Source: CAD feature listing. Evaluate the final solid. Frame: model axes, mm. A direction names the side the tool comes from. Round coordinates to 2 decimals unless told otherwise and drop trailing zeros. Loops run counter-clockwise (first coordinate to the right, second up) from the corner with the lowest first, then second, coordinate; pieces in that order, holes last. Notation, with made-up numbers: M 7.5,63 L 60.5,63 A27 cw 60.5,93 Z; hole C 78.25,54 d8. An arc over 180 degrees is marked long. One line per item, written item: value.
from build123d import *

# Parameters (mm, degrees)
SKETCH1_W           = 20
SKETCH1_H           = 6
BOSS_EXTRUDE1_DEPTH = 30
SKETCH2_W           = 40
SKETCH2_H           = 40
BOSS_EXTRUDE2_DEPTH = 20
FILLET1_R           = 10


with BuildPart() as part:
    # Sketch1 → Boss-Extrude1 (new body)
    with BuildSketch(Plane.XY):
        with Locations((-20, -3)):
            Rectangle(SKETCH1_W, SKETCH1_H)
    extrude(amount=BOSS_EXTRUDE1_DEPTH)

    # Sketch2 → Boss-Extrude2 (add)
    with BuildSketch(Plane.XY):
        with Locations((-10, 14)):
            Rectangle(SKETCH2_W, SKETCH2_H)
    extrude(amount=-BOSS_EXTRUDE2_DEPTH)

    # Fillet1
    # the kernel refuses this fillet: 10 mm, written as the material it adds along each edge
    with BuildSketch(Plane(origin=(-10, 0, 0), x_dir=(0, 1, 0), z_dir=(-1, 0, 0))) as fillet1_piece_1:
        with BuildLine():
            CenterArc((FILLET1_R, -FILLET1_R), FILLET1_R, 90, 90)
            Line((0, -FILLET1_R), (0, 0))
            Line((0, 0), (FILLET1_R, 0))
        make_face()
    extrude(amount=20)
    # the kernel refuses this fillet: 10 mm, written as the material it takes off along each edge
    with BuildSketch(Plane(origin=(10, 34, 25), x_dir=(-1, 0, 0), z_dir=(0, 0, -1))) as fillet1_2_piece_1:
        with BuildLine():
            CenterArc((FILLET1_R, -FILLET1_R), FILLET1_R, 90, 90)
            Line((0, -FILLET1_R), (0, 0))
            Line((0, 0), (FILLET1_R, 0))
        make_face()
    extrude(amount=70, mode=Mode.SUBTRACT)
    with BuildSketch(Plane(origin=(12.912878475, 0, 30), x_dir=(0, 0, -1), z_dir=(-1, 0, 0))) as fillet1_2_piece_2:
        with BuildLine():
            CenterArc((9.16515139, 10), FILLET1_R, 203.578178478, 66.421821522)
            Line((0, 6), (0, 0))
            Line((0, 0), (9.16515139, 0))
        make_face()
    extrude(amount=65.82575695, mode=Mode.SUBTRACT)


solid = part.part
1. Ray query, line 1 (Z direction, x = 4.5, y = 9.5); line 2 (Y direction, x = 8, z = -1.5); line 3 (Y direction, x = -18.5, z = 8). Return the intervals inside material, ascending. Write a range as [from, to].
Report:
line 1: z = [-20, 0]
line 2: y = [-6, 30]
line 3: y = [-6, 0.2]
2. Reachability of faces 1 (the face through (-20, 0, 15)), 2 (the face through (10, 9, -10)), 3 (the face through (-15, -6, 0)), 4 (the face through (-10, -3, 11)), 5 (the face through (-6, 19, 0)) from +Z, -Z, +X, -X, +Y, -Y: full face, straight path, thin tool, end or side. Return the list, or none.
Report:
face 1: +Z, +X, -X, +Y
face 2: +Z, -Z, +X, +Y, -Y
face 3: +Z, -Z, +X, -X, -Y
face 4: +Z, +X, +Y, -Y
face 5: +Z, +X, +Y
3. Section query B-B (y = 2). Return the cut outline in (x, z), and give its area (3 significant figures).
Report:
outline: M -30,-20 L 10,-20 L 10,0 L -10,0 L -10,4 L -30,4 Z
area: 880 mm2
4. Pin query (flat end, axial travel): pin 1 (8.5 mm diameter, centred on x = -18.5, z = 14, fed in from +Y); pin 2 (17.5 mm diameter, centred on y = 3, z = 22, fed in from +X); pin 3 (2 mm diameter, centred on x = 4, y = 12.5, fed in from +Z). Return the tip coordinate at first contact, or that it passes through.
Report:
pin 1: stops at y = 0
pin 2: stops at x = -10
pin 3: stops at z = 0
5. Section query A-A (x = -17). Return the cut outline in (y, z), and give its area (3 significant figures).
Report:
outline: M -6,-20 L 34,-20 L 34,0 L 10,0 A10 cw 0,10 L 0,20.83 A10 ccw -6,30 Z
area: 986 mm2
6. Section query C-C (z = 18). Return the cut outline in (x, y), and give its area (3 significant figures).
Report:
outline: M -30,-6 L -10,-6 L -10,0 L -30,0 Z
area: 120 mm2
7. Section query D-D (y = 22). Return the cut outline in (x, z), and give its area (3 significant figures).
Report:
outline: M -30,-20 L 10,-20 L 10,0 L -30,0 Z
area: 800 mm2
